Could you check a few things on this model? Use its own coordinates, in mm. Face numbers are marked on the shaded views. A direction names the side the tool comes from. Give positions to 0.01 mm unless a question says otherwise; leave off trailing zeros. Loops run counter-clockwise (first coordinate to the right, second up) from the corner with the lowest first, then second, coordinate; pieces in that order, holes last. Notation, with made-up numbers: M 60.5,0.25 L 103.5,0.25 A20 ccw 103.5,31.25 Z; hole C 66,-8.5 d10. An arc over 180 degrees is marked long. Use a Markdown table: item, result. Add a question column.
1) If I drill on line 1 along Z through (x, y) = (6.5, 3); line 2 along Z through (x, y) = (7.5, 7.55) (3 decimals); line 3 along X through (y, z) = (7.35, -7.5) (3 decimals), over which ranges is the centre line in solid material (lowest first)? Write a range as [from, to].
2) Suppose I cut it at B-B on y = 2.75. List the corners of the cut face in (x, z) for me.
3) We'd pull the mould along Z, two halves only. Please class the marked faces 1, 2, 3 and 4: +Z half, -Z half, draft (parallel to the pull), parting line (faces both ways), or undercut.
4) Suppose I cut it at D-D on y = 7.25. List the corners of the cut face in (x, z) for me (3 decimals).
5) Which directions (+Z, -Z, +X, -X, +Y, -Y) give clear straight access to the entire face, cutting with the end or side of a thin tool? Please do the marked faces 5 and 6.
6) Will this pin go through, and if not, where does the flat tip stop? pin 1 Ø3.5 at (x, z) = (7.5, -7.5) entering from -Y.
7) Suppose I cut it at A-A on x = 7.5. List the corners of the cut face in (y, z) for me (3 decimals).
8) Suppose I cut it at C-C on x = 9.25. List the corners of the cut face in (y, z) for me.
```python
from build123d import *

# Parameters (mm, degrees)
SKETCH1_W           = 15
SKETCH1_H           = 15
BOSS_EXTRUDE1_DEPTH = 8
SKETCH3_R           = 2.125
CUT_EXTRUDE3_DEPTH  = 9
CUT_EXTRUDE2_DEPTH  = 6
FILLET1_R           = 2


with BuildPart() as part:
    # Sketch1 → Boss-Extrude1 (new body)
    with BuildSketch(Plane(origin=(0, 0, 0), x_dir=(1, 0, 0), z_dir=(0, 1, 0))):
        with Locations((7.5, 7.5)):
            Rectangle(SKETCH1_W, SKETCH1_H)
    extrude(amount=BOSS_EXTRUDE1_DEPTH)

    # Sketch3 → Cut-Extrude3 (cut, through all)
    with BuildSketch(Plane(origin=(0, 8, 0), x_dir=(1, 0, 0), z_dir=(0, 1, 0))):
        with Locations((7.5, 7.5)):
            Circle(SKETCH3_R)
    extrude(amount=-CUT_EXTRUDE3_DEPTH, mode=Mode.SUBTRACT)

    # Sketch2 → Cut-Extrude2 (cut)
    with BuildSketch(Plane(origin=(0, 0, 0), x_dir=(1, 0, 0), z_dir=(0, 1, 0))):
        Polygon((11.483716857, 7.5), (9.491858429, 10.95), (5.508141571, 10.95), (3.516283143, 7.5), (5.508141571, 4.05), (9.491858429, 4.05), align=None)
    extrude(amount=CUT_EXTRUDE2_DEPTH, mode=Mode.SUBTRACT)

    # Fillet1
    fillet1_edges = [part.edges().sort_by_distance(p)[0] for p in [
        (0, 4, -15),
        (15, 4, -15),
        (15, 4, 0),
        (0, 4, 0),
    ]]
    fillet(fillet1_edges, radius=FILLET1_R)


solid = part.part
```
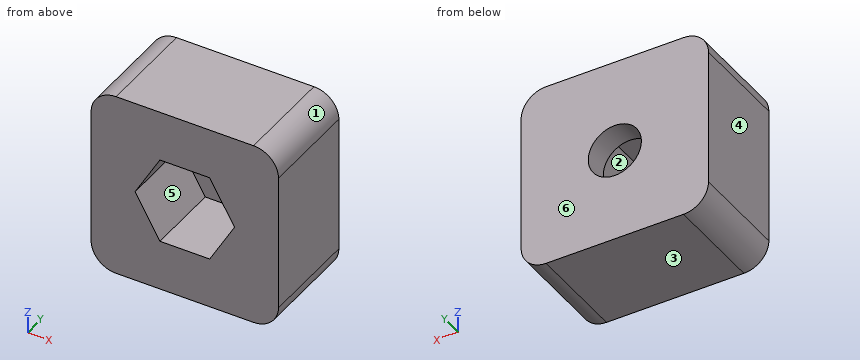
Answer block:
| question | item | result |
|---|---|---|
| 1 | line 1 | z = [-15, -10.95], [-4.05, 0] |
| 1 | line 2 | z = [-15, -9.625], [-5.375, 0] |
| 1 | line 3 | x = [0, 5.375], [9.625, 15] |
| 2 | outline | M 0,-13 A2 ccw 2,-15 L 13,-15 A2 ccw 15,-13 L 15,-2 A2 ccw 13,0 L 2,0 A2 ccw 0,-2 Z; hole M 3.52,-7.5 L 5.51,-10.95 L 9.49,-10.95 L 11.48,-7.5 L 9.49,-4.05 L 5.51,-4.05 Z |
| 3 | face 1 | +Z half |
| 3 | face 2 | undercut |
| 3 | face 3 | -Z half |
| 3 | face 4 | draft |
| 4 | outline | M 0,-13 A2 ccw 2,-15 L 13,-15 A2 ccw 15,-13 L 15,-2 A2 ccw 13,0 L 2,0 A2 ccw 0,-2 Z; hole C 7.5,-7.5 d4.25 |
| 5 | face 5 | -Y |
| 5 | face 6 | +Z, -Z, +X, -X, +Y |
| 6 | pin 1 | passes through |
| 7 | outline | M 0,-15 L 8,-15 L 8,-9.625 L 6,-9.625 L 6,-10.95 L 0,-10.95 Z; M 0,-4.05 L 6,-4.05 L 6,-5.375 L 8,-5.375 L 8,0 L 0,0 Z |
| 8 | outline | M 0,-15 L 8,-15 L 8,-8.71 L 6,-8.71 L 6,-10.95 L 0,-10.95 Z; M 0,-4.05 L 6,-4.05 L 6,-6.29 L 8,-6.29 L 8,0 L 0,0 Z |
